Geometry check sheet. Reference: the model listing, model coordinates, mm. Coordinates: 2 decimals unless noted, no trailing zeros. Loops run counter-clockwise (first coordinate to the right, second up) from the corner with the lowest first, then second, coordinate; pieces in that order, holes last. Notation, with made-up numbers: (-18, 11) - (-1, 11) arc R16 ccw to (-1, 22) - close; hole circle Ø3 at (6.25, 18.5). An arc over 180 degrees is marked (long way). One line per item, written item: value.
from build123d import *

# Parameters (mm, degrees)
SKETCH1_W           = 1.5
SKETCH1_H           = 50
BOSS_EXTRUDE1_DEPTH = 150
SKETCH2_W           = 10
SKETCH2_H           = 82.5
CUT_EXTRUDE1_DEPTH  = 2.5
SKETCH3_W           = 19.117585256
SKETCH3_H           = 37.973569139
POWERCONN_DEPTH     = 2.5
SKETCH4_W           = 10.297175775
SKETCH4_H           = 17.958343038
USBCONN_DEPTH       = 2.5


with BuildPart() as part:
    # Sketch1 → Boss-Extrude1 (new body, symmetric)
    with BuildSketch(Plane(origin=(0, 0, 0), x_dir=(1, 0, 0), z_dir=(0, 1, 0))):
        Rectangle(SKETCH1_W, SKETCH1_H)
    extrude(amount=BOSS_EXTRUDE1_DEPTH, both=True)

    # Sketch2 → Cut-Extrude1 (cut, through all)
    with BuildSketch(Plane.ZY.offset(0.75)):
        with Locations((20, 63.75)):
            Rectangle(SKETCH2_W, SKETCH2_H)
        with Locations((20, -63.75)):
            Rectangle(SKETCH2_W, SKETCH2_H)
    extrude(amount=-CUT_EXTRUDE1_DEPTH, mode=Mode.SUBTRACT)

    # Sketch3 → PowerConn (cut, through all)
    with BuildSketch(Plane.ZY.offset(0.75)):
        with Locations((-7.430305419, -112.401736371)):
            Rectangle(SKETCH3_W, SKETCH3_H)
    extrude(amount=-POWERCONN_DEPTH, mode=Mode.SUBTRACT)

    # Sketch4 → UsbConn (cut, through all)
    with BuildSketch(Plane.ZY.offset(0.75)):
        with Locations((-8.106092581, 115.676720654)):
            Rectangle(SKETCH4_W, SKETCH4_H)
    extrude(amount=-USBCONN_DEPTH, mode=Mode.SUBTRACT)


solid = part.part
(1) Go/stop test with a flat-tipped pin: pin 1 Ø8 at (y, z) = (-103.5, -9.5) entering from -X. Record where the tip stops, or that it passes through.
Reply:
pin 1: through
(2) Cross-section at B-B on x = 0.3. Record the cut outline in (y, z).
Reply:
outline: (-150, -25) - (150, -25) - (150, 25) - (105, 25) - (105, 15) - (22.5, 15) - (22.5, 25) - (-22.5, 25) - (-22.5, 15) - (-105, 15) - (-105, 25) - (-150, 25) - close; hole (-131.39, -16.99) - (-93.41, -16.99) - (-93.41, 2.13) - (-131.39, 2.13) - close; hole (106.7, -13.25) - (124.66, -13.25) - (124.66, -2.96) - (106.7, -2.96) - close
(3) Cross-section at C-C on y = -28.5. Record the cut outline in (x, z), and give its area (3 significant figures).
Reply:
outline: (-0.75, -25) - (0.75, -25) - (0.75, 15) - (-0.75, 15) - close
area: 60.0 mm2
(4) Cross-section at A-A on z = -6.5. Record the cut outline in (x, y), and give its area (3 significant figures).
Reply:
outline: (-0.75, -150) - (0.75, -150) - (0.75, -131.39) - (-0.75, -131.39) - close; (-0.75, -93.41) - (0.75, -93.41) - (0.75, 106.7) - (-0.75, 106.7) - close; (-0.75, 124.66) - (0.75, 124.66) - (0.75, 150) - (-0.75, 150) - close
area: 366 mm2
(5) Material ranges on probe 1 along Y at (x, z) = (-0.55, 19.5); probe 2 along Y at (x, z) = (-0.6, 2); probe 3 along Z at (x, y) = (0.05, 83.5), recorded low to high. Write a range as from..to.
Reply:
probe 1: -150..-105, -22.5..22.5, 105..150
probe 2: -150..-131.39, -93.41..150
probe 3: -25..15
